```python
from build123d import *

# Parameters (mm, degrees)
ESQUISSE2_R             = 3
BOSS_EXTRU_1_DEPTH      = 4
ESQUISSE3_R             = 1.5
ENL_V_MAT_EXTRU_1_DEPTH = 5
CONG_1_R                = 6.5
ESQUISSE4_W             = 4
ESQUISSE4_H             = 12
BOSS_EXTRU_2_DEPTH      = 4
CONG_2_R                = 5
ESQUISSE5_W             = 12
ESQUISSE5_H             = 4
ENL_V_MAT_EXTRU_2_DEPTH = 4


with BuildPart() as part:
    # Esquisse2 → Boss.-Extru.1 (new body)
    with BuildSketch(Plane.XY):
        with BuildLine():
            Line((-199.971644797, -262.478940861), (-196.098548459, -348.633560192))
            ThreePointArc((-196.098548459, -348.633560192), (-8.923258694, -399.900456932), (180.352503917, -357.033575915))
            Line((180.352503917, -357.033575915), (187.115722814, -370.422335012))
            ThreePointArc((187.115722814, -370.422335012), (-9.257880895, -414.896724067), (-203.452244027, -361.707318699))
            Line((-203.452244027, -361.707318699), (-211.920441681, -376.762493353))
            ThreePointArc((-211.920441681, -376.762493353), (-226.337772202, -383.722686379), (-237.858405423, -372.606089933))
            ThreePointArc((-237.858405423, -372.606089933), (-265.801404699, -326.067035455), (-317.01741072, -308.077718418))
            ThreePointArc((-317.01741072, -308.077718418), (-326.924525304, -304.085923492), (-331.133147983, -294.268956483))
            Line((-331.133147983, -294.268956483), (-331.541895531, -264.271741188))
            Line((-331.541895531, -264.271741188), (-199.971644797, -262.478940861))
        make_face()
        with Locations((-317.134447512, -294.078207627)):
            Circle(ESQUISSE2_R, mode=Mode.SUBTRACT)
        with Locations((-212.300150205, -299.974825982)):
            Circle(ESQUISSE2_R, mode=Mode.SUBTRACT)
        with Locations((-224.122616287, -369.899044157)):
            Circle(ESQUISSE2_R, mode=Mode.SUBTRACT)
    extrude(amount=BOSS_EXTRU_1_DEPTH)

    # Esquisse3 → Enlèv. mat.-Extru.1 (cut, through all)
    with BuildSketch(Plane.XY.offset(4)):
        with Locations((172.9434239, -368.980788294)):
            Circle(ESQUISSE3_R)
        with BuildLine():
            Line((169.760416098, -362.18973084), (162.877223829, -362.18973084))
            Line((162.877223829, -362.18973084), (180.965097343, -354.152116582))
            Line((180.965097343, -354.152116582), (180.352503917, -357.033575915))
            Line((180.352503917, -357.033575915), (187.115722814, -370.422335012))
            Line((187.115722814, -370.422335012), (190.286834204, -373.47465723))
            Line((190.286834204, -373.47465723), (174.853495029, -378.475059123))
            Line((174.853495029, -378.475059123), (176.126431702, -375.771845747))
            ThreePointArc((176.126431702, -375.771845747), (179.734481353, -365.797780492), (169.760416098, -362.18973084))
        make_face()
    extrude(amount=-ENL_V_MAT_EXTRU_1_DEPTH, mode=Mode.SUBTRACT)

    # Congé1
    cong_1_edges = [part.edges().sort_by_distance(p)[0] for p in [
        (-203.452244027, -361.707318699, 2),
        (-196.098548459, -348.633560192, 2),
    ]]
    fillet(cong_1_edges, radius=CONG_1_R)

    # Esquisse4 → Boss.-Extru.2 (add)
    with BuildSketch(Plane.XY.offset(4)):
        Polygon((-211.920441681, -376.762493353), (-223.686354588, -397.680506965), (-245.4759521, -385.424347686), (-237.96555462, -372.071996878), (-225.374330656, -376.762493353), align=None)
        Polygon((-238.339917634, -385.996197397), (-227.880910828, -391.879153851), (-225.919925343, -388.392818249), (-236.378932149, -382.509861795), align=None, mode=Mode.SUBTRACT)
        Polygon((-316.348629052, -308.074922938), (-340.348629052, -308.074922938), (-340.348629052, -283.074922938), (-331.285679934, -283.074922938), align=None)
        with Locations((-335.348629052, -295.574922938)):
            Rectangle(ESQUISSE4_W, ESQUISSE4_H, mode=Mode.SUBTRACT)
    extrude(amount=-BOSS_EXTRU_2_DEPTH)

    # Congé2
    cong_2_edges = [part.edges().sort_by_distance(p)[0] for p in [
        (-340.348629052, -308.074922938, 2),
        (-340.348629052, -283.074922938, 2),
        (-223.686354588, -397.680506965, 2),
        (-245.4759521, -385.424347686, 2),
        (-237.96555462, -372.071996878, 2),
    ]]
    fillet(cong_2_edges, radius=CONG_2_R)

    # Esquisse5 → Enlèv. mat.-Extru.2 (cut)
    with BuildSketch(Plane.XY.offset(4)):
        with Locations((-234.450045065, -274.867921079)):
            Rectangle(ESQUISSE5_W, ESQUISSE5_H)
    extrude(amount=-ENL_V_MAT_EXTRU_2_DEPTH, mode=Mode.SUBTRACT)


solid = part.part
```
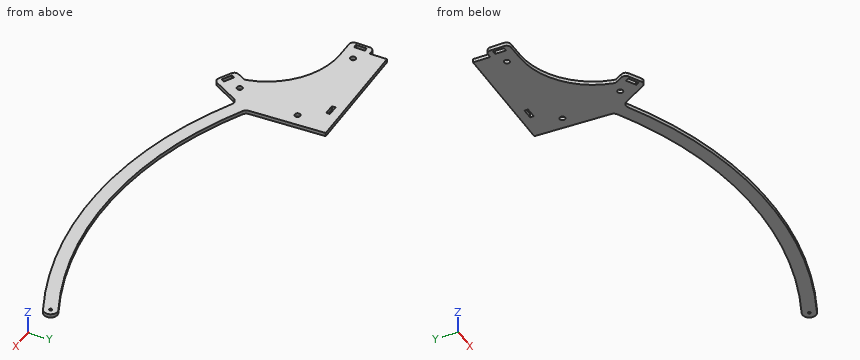
Design review of the part built by this model. Coordinates are the model's own, in mm. Give positions to 0.01 mm unless a question says otherwise; leave off trailing zeros. Order: outer loops, then holes, each group sorted by start corner. A loop starts at its lowest first (then second) coordinate and runs counter-clockwise, first axis right, second up. Notation, with made-up numbers: (-38, 6.25) - (-22, 6.25) arc R8 cw to (-22, 20.25) - close; hole circle Ø11 at (22, 66.5). An arc over 180 degrees is marked (long way). Use a Markdown table: item, result. Add a question column.
(1) Add section A-A on x = -104.5. Give the boundary of the cut face in (y, z), then the cut area to 3 significant figures.
(2) Add section B-B on y = -330. Give the boundary of the cut face in (x, z).
(3) Clearance check with flat-ended pins moving along their axes: P1, Ø1, axis at x = -149, z = 3, coming from the +Y side; P2, Ø2, axis at x = -233.5, z = 2.5, coming from the -Y side; P3, Ø1.2, axis at x = -326, z = 3, coming from the -Y side. State where each tip first meets the part, or that it passes through.
(4) Add section C-C on z = 1.15. Give the number of separate pieces and of enclosed holes in the cut face, then the cut area to 3 significant figures.
(5) Wall thickness on probe 1 along Y at (x, z) = (-226.5, 2.8); probe 2 along X at (y, z) = (-298, 0.8); probe 3 along Y at (x, z) = (-201.5, 2.1): over which ranges is each line inside the solid? List them lowest first. Write a range as [from, to].
Report:
| question | item | result |
|---|---|---|
| 1 | outline | (-401.63, 0) - (-386.11, 0) - (-386.11, 4) - (-401.63, 4) - close |
| 1 | area | 62.1 mm² |
| 2 | outline | (-261.33, 0) - (-196.94, 0) - (-196.94, 4) - (-261.33, 4) - close |
| 3 | P1 | stops at y = -371.01 |
| 3 | P2 | stops at y = -392.72 |
| 3 | P3 | stops at y = -308.07 |
| 4 | separate pieces | 1 |
| 4 | enclosed holes | 7 |
| 4 | area | 16,100 mm² |
| 5 | probe 1 | y = [-395.79, -389.42], [-388.07, -371.73], [-368.07, -262.84] |
| 5 | probe 2 | x = [-340.35, -337.35], [-333.35, -214.56], [-210.04, -198.37] |
| 5 | probe 3 | y = [-364.04, -262.5] |
